from build123d import *

# Parameters (mm, degrees)
F0_W     = 254
F0_H     = 19.05
F1_DEPTH = 50.8
F2_DEPTH = 50.8
F4_W     = 19.05
F4_H     = 19.05
F4_R     = 6.35
F5_DEPTH = 127
F7_DEPTH = 50.8


# Not quite as in the source:
# - a feature names something its author has since deleted; it is built from what else it names


with BuildPart() as f1:
    # F0 (on Front) → F1 (new body)
    with BuildSketch(Plane.XZ):
        with Locations((0, 111.1250000177)):
            Rectangle(F0_W, F0_H)
    extrude(amount=F1_DEPTH)

    # F0 (on Front) → F2 (join, through all)
    with BuildSketch(Plane.XZ):
        with BuildLine():
            Line((127, 82.5500000177), (127, 101.6000000177))
            Line((127, 101.6000000177), (-127, 101.6000000177))
            Line((-127, 101.6000000177), (-127, 12.7000000177))
            ThreePointArc((-127, 12.7000000177), (-69.8499999823, -44.45), (-127, -101.6000000177))
            Line((-127, -101.6000000177), (-127, -127.0000000177))
            Line((-127, -127.0000000177), (-101.6, -127.0000000177))
            Line((-101.6, -127.0000000177), (88.9, -127.0000000177))
            Line((88.9, -127.0000000177), (127, -127.0000000177))
            Line((127, -127.0000000177), (127, -101.6000000177))
            ThreePointArc((127, -101.6000000177), (75.1661658016, -83.0433945651), (46.8866745136, -35.8060751437))
            ThreePointArc((46.8866745136, -35.8060751437), (45.7784438509, -28.4901624232), (45.3368966297, -21.1039732713))
            ThreePointArc((45.3368966297, -21.1039732713), (67.248156143, 45.6292415321), (127, 82.5500000177))
        make_face()
    extrude(amount=F2_DEPTH)

    # F3: F1 across face


with BuildPart() as f1_1:
    add(f1.part)
    add(f1.part.mirror(Plane(origin=(-11.712184673, 0, 3.7973817679), x_dir=(1, 0, 0), z_dir=(0, 1, 0))))

    # F4 (on Top) → F5 (cut)
    with BuildSketch(Plane.XY):
        with Locations((82.55, 0)):
            Rectangle(F4_W, F4_H)
        with Locations((107.95, 25.4)):
            Circle(F4_R)
    extrude(amount=F5_DEPTH, mode=Mode.SUBTRACT)



with BuildPart() as f7:
    # F0 (on Front) → F7 (new body)
    with BuildSketch(Plane.XZ):
        with BuildLine():
            Line((-127, 12.7000000177), (-127, 101.6000000177))
            add(Edge.make_bspline(
                [(-127, 101.6000000177), (-143.1548670141, 101.1279175586), (-178.3487321582, 100.5000750149), (-235.9685551739, 104.8555928403), (-254, 107.5927615166)],
                knots=[0, 0, 0, 0, 0.4585605976, 1, 1, 1, 1], degree=3))
            ThreePointArc((-254, 107.5927615166), (-268.9111687536, 100.3097468732), (-265.0851011276, 84.1621011496))
            add(Edge.make_bspline(
                [(-265.0851011276, 84.1621011496), (-258.982913814, 78.2797981737), (-242.4670319791, 62.3590460812), (-161.6065585576, 21.8898515634), (-136.6674442933, 15.2672145631), (-127, 12.7000000177)],
                knots=[0, 0, 0, 0, 0.2640715847, 0.7147231864, 1, 1, 1, 1], degree=3))
        make_face()
    extrude(amount=F7_DEPTH)


with BuildPart() as f1_2:
    add(f1_1.part)

    add(f7.part)  # F6 merges F7
    # F6: F7 across plane
    add(f7.part.mirror(Plane.XZ))


solid = f1_2.part
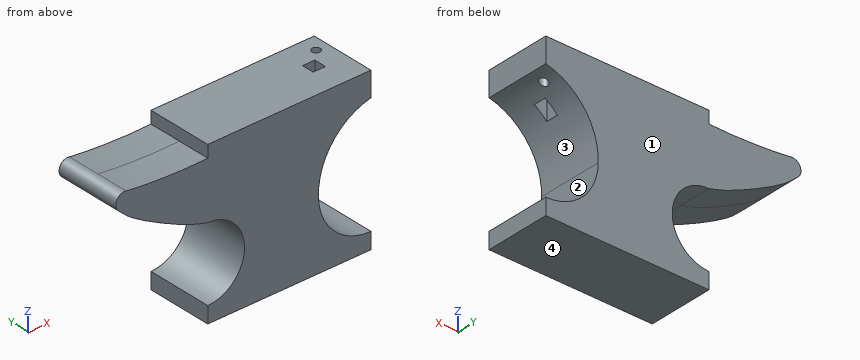
Verification items for the finished model (mm, model axes). Face numbers are marked on the shaded views. Give positions to 0.01 mm unless a question says otherwise; leave off trailing zeros. Order: outer loops, then holes, each group sorted by start corner. A loop starts at its lowest first (then second) coordinate and runs counter-clockwise, first axis right, second up. Notation, with made-up numbers: M -7.75,4 L 44.25,4 A25 cw 44.25,43 Z; hole C 12.25,29.25 d11. An arc over 180 degrees is marked long. Answer as a JSON object with one key per item and string values. Group by question number.
1) Scan lines: line 1 along Y through (x, z) = (107.95, 92.5); line 2 along X through (y, z) = (25, 86); line 3 along Z through (x, y) = (81.5, 35.5). Record each from-to range of solid material in increasing order. Write a range as [from, to].
2) Cross-section at A-A (x = 107.95). Enter the section's corners in (y, z).
3) Mould release check, pull along Z, two halves, no side actions. Record for the marked faces 1, 2, 3 and 4: released by +Z, released by -Z, zero draft, split by the parting line, or undercut.
4) Cross-section at B-B (z = -44.45). Enter the section's corners in (x, y), then the cut area to 3 significant figures.
5) Depth check by flat-ended pin: pin 1 Ø4 at (x, y) = (-155, -24.5) entering from +Z; pin 2 Ø7.5 at (y, z) = (-18.5, -119.5) entering from -X; pin 3 Ø9.5 at (y, z) = (3, 90.5) entering from -X; pin 4 Ø8 at (y, z) = (-35, -37) entering from -X. Enter the tip coordinate at first touch or a pass-through.
Result sheet:
{
 "1": {"line 1": "y = [-50.8, 19.05], [31.75, 50.8]", "line 2": "x = [-267, 101.61], [114.29, 127]", "line 3": "z = [-127, -87.75], [60.4, 120.65]"},
 "2": {"outline": "M -50.8,-127 L 50.8,-127 L 50.8,-99.35 L -50.8,-99.35 Z; M -50.8,76.64 L 19.05,76.64 L 19.05,120.65 L -50.8,120.65 Z; M 31.75,76.64 L 50.8,76.64 L 50.8,120.65 L 31.75,120.65 Z"},
 "3": {"face 1": "zero draft", "face 2": "undercut", "face 3": "undercut", "face 4": "released by -Z"},
 "4": {"outline": "M -69.85,-50.8 L 49.1,-50.8 L 49.1,50.8 L -69.85,50.8 Z", "area": "12,100 mm2"},
 "5": {"pin 1": "stops at z = 101.14", "pin 2": "stops at x = -127", "pin 3": "stops at x = -270.19", "pin 4": "stops at x = -71.01"}
}
